```python
from build123d import *

# Parameters (mm, degrees)
PAD001_DEPTH          = 1.2
SKETCH002_R           = 3
PAD002_DEPTH          = 3
SKETCH003_R           = 0.8
POCKET_DEPTH          = 5
CLONE_PLACEMENT_ANGLE = 180


with BuildPart() as part:
    # Sketch001 → Pad001 (new body)
    with BuildSketch(Plane.XY):
        with BuildLine():
            ThreePointArc((-47.75, 5), (-52.75, 0), (-47.75, -5))
            Line((-43, -5), (-47.75, -5))
            Line((-43, 5), (-43, -5))
            Line((-47.75, 5), (-43, 5))
        make_face()
    extrude(amount=PAD001_DEPTH)

    # Sketch002 → Pad002 (new body)
    with BuildSketch(Plane.XY.offset(1.2)):
        with Locations((-47.75, 0)):
            Circle(SKETCH002_R)
    extrude(amount=PAD002_DEPTH)

    # Sketch003 → Pocket (cut)
    with BuildSketch(Plane.XY.offset(4.2)):
        with Locations((-47.75, 0)):
            Circle(SKETCH003_R)
    extrude(amount=-POCKET_DEPTH, mode=Mode.SUBTRACT)


with BuildPart() as part_1:
    # Clone placement: moved
    add(part.part.moved(Location((16, 0, 0))).rotate(Axis((16, 0, 0), (0, 0, 1)), CLONE_PLACEMENT_ANGLE))


solid = part_1.part
```
Model file for the job. Use its own axes, mm. A direction names the side the tool comes from. Give positions to 0.01 mm unless a question says otherwise; leave off trailing zeros. Loops run counter-clockwise (first coordinate to the right, second up) from the corner with the lowest first, then second, coordinate; pieces in that order, holes last. Notation, with made-up numbers: M 22,66 L 43,66 A25 ccw 43,96 Z; hole C 84.5,-8.75 d11. An arc over 180 degrees is marked long. Use one line per item in the form item = value.
Item 1: Slice it at D-D on z = 1.7. List the corners of the cut face in (x, y).
Filled in:
outline = C 63.75,0 d6; hole C 63.75,0 d1.6
Item 2: Two-plate mould, pull along Y, no slides. Class faces 1 (the cylindrical face through (62.987, -0.24, 2.129)), 2 (the flat face through (61, -5, 1)), 3 (the flat face through (61, 5, 1)): released by +Y, released by -Y, zero draft, split by the parting line, or undercut.
Filled in:
face_1 = undercut
face_2 = released by -Y
face_3 = released by +Y
Item 3: Slice it at C-C on y = -2.5. List the corners of the cut face in (x, z), and give its area (3 significant figures).
Filled in:
outline = M 59,0 L 68.08,0 L 68.08,1.2 L 65.41,1.2 L 65.41,4.2 L 62.09,4.2 L 62.09,1.2 L 59,1.2 Z
area = 20.8 mm^2
Item 4: Which spindle directions (+Z, -Z, +X, -X, +Y, -Y) get a long thin tool onto all of the face, cutting with end or side? Do faces 4 (the flat face through (64, 1, 0)), 5 (the cylindrical face through (66.131, 1.825, 2.679)). Say none if no direction does.
Filled in:
face_4 = -Z, +X, -X, +Y, -Y
face_5 = +Z
Item 5: Slice it at B-B on x = 64. List the corners of the cut face in (y, z).
Filled in:
outline = M -4.99,0 L -0.76,0 L -0.76,4.2 L -2.99,4.2 L -2.99,1.2 L -4.99,1.2 Z; M 0.76,0 L 4.99,0 L 4.99,1.2 L 2.99,1.2 L 2.99,4.2 L 0.76,4.2 Z
Item 6: Flat gauge pin, fed straight in: pin 1 Ø1 at (x, y) = (63.75, 0) entering from -Z. Where does the tip first touch, or does it go through?
Filled in:
pin_1 = through
Item 7: Slice it at A-A on y = 0. List the corners of the cut face in (x, z), and give its area (3 significant figures).
Filled in:
outline = M 59,0 L 62.95,0 L 62.95,4.2 L 60.75,4.2 L 60.75,1.2 L 59,1.2 Z; M 64.55,0 L 68.75,0 L 68.75,1.2 L 66.75,1.2 L 66.75,4.2 L 64.55,4.2 Z
area = 23.0 mm^2
Item 8: Drill centre lines: L1, parallel to Y at x = 63.75, z = 3.2; L2, parallel to X at y = 0, z = 2.8; L3, parallel to Z at x = 67.5, y = -2. Where is each one in solid material? Low to high.
Filled in:
L1 = -3 to -0.8, 0.8 to 3
L2 = 60.75 to 62.95, 64.55 to 66.75
L3 = 0 to 1.2
